from build123d import *

# Parameters (mm, degrees)
ESBO_O1_R                = 11
RESSALTO_EXTRUS_O1_DEPTH = 2.38125
ESBO_O2_R                = 11
ESBO_O2_R_2              = 10
CORTE_EXTRUS_O1_DEPTH    = 0.5
CORTE_EXTRUS_O3_DEPTH    = 17.269032124


with BuildPart() as part:
    # Esboço1 → Ressalto-extrusão1 (new, symmetric)
    with BuildSketch(Plane(origin=(0, 0, 0), x_dir=(1, 0, 0), z_dir=(0, 1, 0))):
        with Locations(Location((0, 0, 0), (0, 0, 90))):
            Circle(ESBO_O1_R)
    extrude(amount=RESSALTO_EXTRUS_O1_DEPTH, both=True)

    # Esboço2 → Corte-extrusão1 (cut, symmetric)
    with BuildSketch(Plane(origin=(0, 0, 0), x_dir=(1, 0, 0), z_dir=(0, 1, 0))):
        with Locations(Location((0, 0, 0), (0, 0, 90))):
            Circle(ESBO_O2_R)
        with Locations(Location((0, 0, 0), (0, 0, 270))):
            Circle(ESBO_O2_R_2, mode=Mode.SUBTRACT)
    extrude(amount=CORTE_EXTRUS_O1_DEPTH, both=True, mode=Mode.SUBTRACT)

    # Esboço4 → Corte-extrusão3 (cut, through all)
    with BuildSketch(Plane(origin=(0, 2.38125, 0), x_dir=(1, 0, 0), z_dir=(0, 1, 0))):
        with BuildLine():
            Line((-2.246839856, 0.491640786), (-0.697646517, -2.191640786))
            ThreePointArc((-0.697646517, -2.191640786), (0, -2.3), (0.697646517, -2.191640786))
            Line((0.697646517, -2.191640786), (2.246839856, 0.491640786))
            ThreePointArc((2.246839856, 0.491640786), (1.991858429, 1.15), (1.549193338, 1.7))
            Line((1.549193338, 1.7), (-1.549193338, 1.7))
            ThreePointArc((-1.549193338, 1.7), (-1.991858429, 1.15), (-2.246839856, 0.491640786))
        make_face()
    extrude(amount=-CORTE_EXTRUS_O3_DEPTH, mode=Mode.SUBTRACT)


solid = part.part
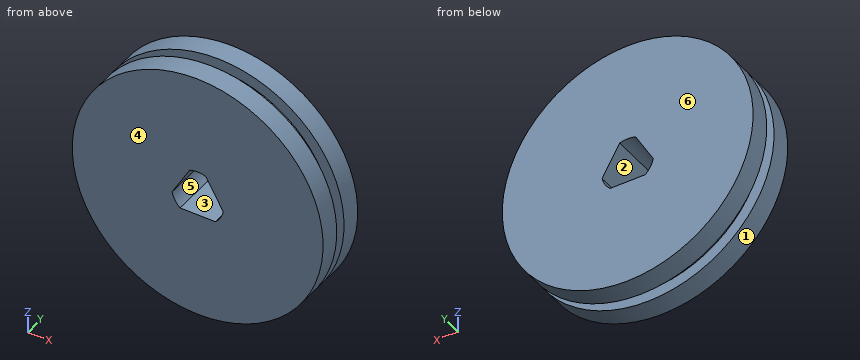
Verification items for the finished model (mm, model axes). Face numbers are marked on the shaded views. A direction names the side the tool comes from. Coordinates: 2 decimals unless noted, no trailing zeros. Order: outer loops, then holes, each group sorted by start corner. A loop starts at its lowest first (then second) coordinate and runs counter-clockwise, first axis right, second up.
1. Sectioned sample at C-C, the plane z = -0.75. Record the cut outline in (x, y), and give its area (3 significant figures).
Results found:
outline: (-10.97, -2.38) - (-2.17, -2.38) - (-2.17, 2.38) - (-10.97, 2.38) - (-10.97, 0.5) - (-9.97, 0.5) - (-9.97, -0.5) - (-10.97, -0.5) - close; (2.17, -2.38) - (10.97, -2.38) - (10.97, -0.5) - (9.97, -0.5) - (9.97, 0.5) - (10.97, 0.5) - (10.97, 2.38) - (2.17, 2.38) - close
area: 81.8 mm2
2. Sectioned sample at B-B, the plane y = 1.2. Record the cut outline in (x, z), and give its area (3 significant figures).
Results found:
outline: circle Ø22 at (0, 0); hole (-2.25, -0.49) arc R2.3 ccw to (-1.55, -1.7) - (1.55, -1.7) arc R2.3 ccw to (2.25, -0.49) - (0.7, 2.19) arc R2.3 ccw to (-0.7, 2.19) - close
area: 367 mm2
3. Scan lines: line 1 (Y direction, x = -4, z = -10); line 2 (X direction, y = 0.75, z = 0); line 3 (X direction, y = 1.8, z = -0.5) (3 decimals). Record each from-to range of solid material in increasing order.
Results found:
line 1: y = -2.38 to -0.5, 0.5 to 2.38
line 2: x = -11 to -1.96, 1.96 to 11
line 3: x = -10.989 to -2.245, 2.245 to 10.989
4. Sectioned sample at A-A, the plane x = 0. Record the cut outline in (y, z).
Results found:
outline: (-2.38, -11) - (-0.5, -11) - (-0.5, -10) - (0.5, -10) - (0.5, -11) - (2.38, -11) - (2.38, -1.7) - (-2.38, -1.7) - close; (-2.38, 2.3) - (2.38, 2.3) - (2.38, 11) - (0.5, 11) - (0.5, 10) - (-0.5, 10) - (-0.5, 11) - (-2.38, 11) - close
5. Set-up check for the marked faces 5 and 6: record each of +Z, -Z, +X, -X, +Y, -Y from which the full face is reachable in a straight line by a thin tool's end or side.
Results found:
face 5: +Y, -Y
face 6: +Z, -Z, +X, -X, +Y
6. Sectioned sample at D-D, the plane x = -7. Record the cut outline in (y, z), and give its area (3 significant figures).
Results found:
outline: (-2.38, -8.49) - (-0.5, -8.49) - (-0.5, -7.14) - (0.5, -7.14) - (0.5, -8.49) - (2.38, -8.49) - (2.38, 8.49) - (0.5, 8.49) - (0.5, 7.14) - (-0.5, 7.14) - (-0.5, 8.49) - (-2.38, 8.49) - close
area: 78.1 mm2
7. Go/stop test with flat-tipped pins: pin 1 Ø1 at (x, y) = (-2.5, -2) entering from -Z; pin 2 Ø1 at (y, z) = (0.5, 2) entering from -X; pin 3 Ø1.5 at (x, y) = (5.5, -0.5) entering from -Z. Record where each tip stops, or that it passes through.
Results found:
pin 1: stops at z = -10.82
pin 2: stops at x = -10.9
pin 3: stops at z = -9.92
8. Release check for a two-part mould opening along X. For the marked faces 1, 2, 3 and 4 record: +X half, -X half, draft (parallel to the pull), parting line (faces both ways), or undercut.
Results found:
face 1: parting line
face 2: undercut
face 3: undercut
face 4: draft
